```python
from build123d import *

# Parameters (mm, degrees)
F0_W     = 26
F0_H     = 7
F2_DEPTH = 0.15
F1_R     = 2
F3_DEPTH = 0.1


with BuildPart() as f2:
    # F0 (on Top) → F2 (new body)
    with BuildSketch(Plane.XY):
        Rectangle(F0_W, F0_H)
    extrude(amount=-F2_DEPTH)

    # F1 (on Top) → F3 (join)
    with BuildSketch(Plane.XY):
        with Locations((-10, 0)):
            Circle(F1_R)
    extrude(amount=F3_DEPTH)


solid = f2.part
```
Work out the finished part from the listing and answer in its coordinate system (mm). Coordinates: 2 decimals unless noted, no trailing zeros. Write each loop counter-clockwise with the first axis right and the second up, starting at its lowest first coordinate (ties: lowest second). Pieces come first, ordered by that corner, then holes. Notation, with made-up numbers: (81.5, 76.25) - (111.5, 76.25) arc R28 cw to (111.5, 99.25) - close; hole circle Ø1 at (27.5, -37). An arc over 180 degrees is marked (long way). Answer as a JSON object with one key per item and string values.
Q1. Find section A-A (x = -10). Write down the section's boundary in (y, z), plus the area to 3 significant figures.
Results list:
{"outline": "(-3.5, -0.15) - (3.5, -0.15) - (3.5, 0) - (2, 0) - (2, 0.1) - (-2, 0.1) - (-2, 0) - (-3.5, 0) - close", "area": "1.45 mm^2"}
Q2. Given pin 1 Ø4 at (x, y) = (2.5, -2.5) entering from +Z, flat-ended and moving along its own axis, determine where the tip first touches the part or whether it passes through.
Results list:
{"pin 1": "stops at z = 0"}
Q3. Find section B-B (y = 0). Write down the section's boundary in (x, z).
Results list:
{"outline": "(-13, -0.15) - (13, -0.15) - (13, 0) - (-8, 0) - (-8, 0.1) - (-12, 0.1) - (-12, 0) - (-13, 0) - close"}
Q4. Find section C-C (z = 0.05). Write down the section's boundary in (x, y).
Results list:
{"outline": "circle Ø4 at (-10, 0)"}
Q5. Consider L1, parallel to Z at x = 8.5, y = -1.5; L2, parallel to Y at x = -8.5, z = 0.05; L3, parallel to X at y = -1.25, z = 0.05. Determine where each line is inside the solid, lowest interval first. Write a range as from..to.
Results list:
{"L1": "z = -0.15..0", "L2": "y = -1.32..1.32", "L3": "x = -11.56..-8.44"}
Q6. Find section D-D (y = 3). Write down the section's boundary in (x, z), plus the area to 3 significant figures.
Results list:
{"outline": "(-13, -0.15) - (13, -0.15) - (13, 0) - (-13, 0) - close", "area": "3.90 mm^2"}
